```python
from build123d import *

# Parameters (mm, degrees)
BOSS_EXTRUDE2_DEPTH = 40
SKETCH3_R           = 6
SKETCH3_R_2         = 2.1
SKETCH3_R_3         = 2
CUT_EXTRUDE1_DEPTH  = 71.710678119
SKETCH4_R           = 2
CUT_EXTRUDE3_DEPTH  = 10
RIB3_REACH          = 66.226
SKETCH7_WALL_W      = 151.665529222
SKETCH7_WALL_H      = 10
SKETCH8_W           = 7
SKETCH8_H           = 40
CUT_EXTRUDE4_DEPTH  = 70.641941386
SKETCH9_R           = 3.25
CUT_EXTRUDE5_DEPTH  = 67.400301204
SKETCH10_R          = 2
CUT_EXTRUDE6_DEPTH  = 67.400301204


with BuildPart() as part:
    # Sketch1 → Boss-Extrude2 (new body)
    with BuildSketch(Plane(origin=(0, 0, 0), x_dir=(1, 0, 0), z_dir=(0, 1, 0))):
        Polygon((0, 0), (50, 0), (50, 5), (5, 5), (5, 35), (0, 35), align=None)
    extrude(amount=BOSS_EXTRUDE2_DEPTH)

    # Sketch3 → Cut-Extrude1 (cut, through all)
    with BuildSketch(Plane(origin=(0, 0, -5), x_dir=(-1, 0, 0), z_dir=(0, 0, -1))):
        with Locations((-35, 12)):
            Circle(SKETCH3_R)
        with Locations((-35, 23)):
            Circle(SKETCH3_R_2)
        with Locations((-44.2, 32)):
            Circle(SKETCH3_R_3)
        with Locations((-25.8, 32)):
            Circle(SKETCH3_R_3)
    extrude(amount=-CUT_EXTRUDE1_DEPTH, mode=Mode.SUBTRACT)

    # Sketch4 → Cut-Extrude3 (cut)
    with BuildSketch(Plane(origin=(5, 0, 0), x_dir=(0, 0, -1), z_dir=(1, 0, 0))):
        with Locations((12, 32)):
            Circle(SKETCH4_R)
        with Locations((12, 8)):
            Circle(SKETCH4_R)
    extrude(amount=-CUT_EXTRUDE3_DEPTH, mode=Mode.SUBTRACT)

    # Sketch7 wall → Rib3 (add, up to next)
    with BuildSketch(Plane(origin=(12.5, 20, -12.5), x_dir=(0.707106781187, 0, 0.707106781187), z_dir=(0.707106781187, 0, -0.707106781187)), mode=Mode.PRIVATE) as rib3_sk1:
        Rectangle(SKETCH7_WALL_W, SKETCH7_WALL_H)
    rib3_tool1 = extrude(rib3_sk1.sketch, amount=-RIB3_REACH, mode=Mode.PRIVATE) - part.part
    add(rib3_tool1.solids().sort_by_distance((12.5, 20, -12.5))[0])

    # Sketch8 → Cut-Extrude4 (cut, through all)
    with BuildSketch(Plane(origin=(5, 0, 0), x_dir=(0, 0, -1), z_dir=(1, 0, 0))):
        with Locations((31.5, 20)):
            Rectangle(SKETCH8_W, SKETCH8_H)
    extrude(amount=-CUT_EXTRUDE4_DEPTH, mode=Mode.SUBTRACT)

    # Sketch9 → Cut-Extrude5 (cut, through all)
    with BuildSketch(Plane(origin=(5, 0, 0), x_dir=(0, 0, -1), z_dir=(1, 0, 0))):
        with Locations((20, 20)):
            Circle(SKETCH9_R)
    extrude(amount=CUT_EXTRUDE5_DEPTH, mode=Mode.SUBTRACT)

    # Sketch10 → Cut-Extrude6 (cut, through all)
    with BuildSketch(Plane(origin=(5, 0, 0), x_dir=(0, 0, -1), z_dir=(1, 0, 0))):
        with Locations((20, 20)):
            Circle(SKETCH10_R)
    extrude(amount=-CUT_EXTRUDE6_DEPTH, mode=Mode.SUBTRACT)


solid = part.part
```
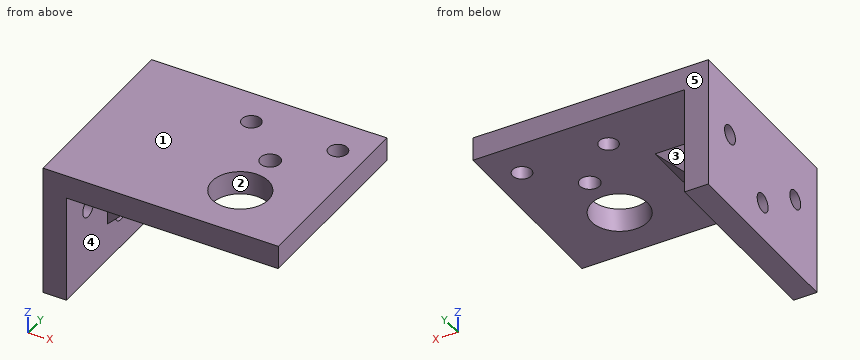
Verification items for the finished model (mm, model axes). Face numbers are marked on the shaded views. A direction names the side the tool comes from. Coordinates: 2 decimals unless noted, no trailing zeros. Loops run counter-clockwise (first coordinate to the right, second up) from the corner with the lowest first, then second, coordinate; pieces in that order, holes last. Notation, with made-up numbers: (0, -17.5) - (14, -17.5) arc R18 cw to (14, -8.5) - close; hole circle Ø11 at (-39, 44). An arc over 180 degrees is marked (long way). Return JSON: item names as keys, results as strings.
1. Go/stop test with flat-tipped pins: pin 1 (6.5 mm diameter, centred on y = 8, z = -12, fed in from +X); pin 2 (7 mm diameter, centred on y = 17, z = -19.5, fed in from +X); pin 3 (4.5 mm diameter, centred on x = 9.5, z = -13, fed in from +Y). Record where each tip stops, or that it passes through.
Established:
{"pin 1": "stops at x = 5", "pin 2": "stops at x = 9", "pin 3": "stops at y = 25"}
2. Section check A-A, the plane x = 44.2. Record the boundary of the cut face in (y, z).
Established:
{"outline": "(0, -5) - (30, -5) - (30, 0) - (0, 0) - close; (34, -5) - (40, -5) - (40, 0) - (34, 0) - close"}
3. Section check D-D, the plane x = 35. Record the boundary of the cut face in (y, z), then the cut area to 3 significant figures.
Established:
{"outline": "(0, -5) - (6, -5) - (6, 0) - (0, 0) - close; (18, -5) - (20.9, -5) - (20.9, 0) - (18, 0) - close; (25.1, -5) - (40, -5) - (40, 0) - (25.1, 0) - close", "area": "119 mm2"}
4. Section check B-B, the plane z = -12. Record the boundary of the cut face in (x, y), then the cut area to 3 significant figures.
Established:
{"outline": "(0, 0) - (5, 0) - (5, 6) - (0, 6) - close; (0, 10) - (5, 10) - (5, 15) - (13, 15) - (13, 25) - (5, 25) - (5, 30) - (0, 30) - close; (0, 34) - (5, 34) - (5, 40) - (0, 40) - close", "area": "240 mm2"}
5. Thickness scan on L1, parallel to Y at x = 35, z = -3.4; L2, parallel to Z at x = 39, y = 5; L3, parallel to X at y = 32, z = -21. Record the ranges inside material, lowest first.
Established:
{"L1": "y = 0 to 6, 18 to 20.9, 25.1 to 40", "L2": "z = -5 to 0", "L3": "x = 0 to 5"}
6. Tool access check on the marked faces 4 and 5. Record the directions out of +Z, -Z, +X, -X, +Y, -Y that give a thin tool (end or side, any length) a straight path to the whole face; none if there is none.
Established:
{"face 4": "-Z, +X", "face 5": "+Z, -Z, +X, -X, +Y"}
7. Section check C-C, the plane y = 32. Record the boundary of the cut face in (x, z).
Established:
{"outline": "(0, -28) - (5, -28) - (5, -14) - (0, -14) - close; (0, -10) - (5, -10) - (5, -5) - (23.8, -5) - (23.8, 0) - (0, 0) - close; (27.8, -5) - (42.2, -5) - (42.2, 0) - (27.8, 0) - close; (46.2, -5) - (50, -5) - (50, 0) - (46.2, 0) - close"}
8. Mould release check, pull along Y, two halves, no side actions. Record for the marked faces 1, 2 and 3: +Y half, -Y half, draft (parallel to the pull), parting line (faces both ways), or undercut.
Established:
{"face 1": "draft", "face 2": "undercut", "face 3": "+Y half"}
